```python
from build123d import *

# Parameters (mm, degrees)
SKETCH1_W            = 10.5
SKETCH1_H            = 6
BOSS_EXTRUDE1_DEPTH  = 7.07
SKETCH3_W            = 8.6
SKETCH3_H            = 1.8
CUT_EXTRUDE2_DEPTH   = 17
SKETCH4_W            = 10.5
SKETCH4_H            = 6
BOSS_EXTRUDE2_DEPTH  = 7.07
SKETCH5_W            = 4
SKETCH5_H            = 1.8
CUT_EXTRUDE3_DEPTH   = 19
FILLET1_R            = 12
FILLET2_R            = 12
SKETCH19_W           = 10.5
SKETCH19_H           = 11
SKETCH19_W_2         = 4
SKETCH19_H_2         = 1.8
BOSS_EXTRUDE8_DEPTH  = 15
CUT_EXTRUDE8_DEPTH   = 14.5
SKETCH21_W           = 10.5
SKETCH21_H           = 15
BOSS_EXTRUDE9_DEPTH  = 1
CUT_EXTRUDE10_DEPTH  = 15
FILLET6_R            = 2
FILLET12_R           = 2
BOSS_EXTRUDE15_DEPTH = 13
FILLET15_R           = 2
FILLET16_R           = 2
FILLET17_R           = 2


with BuildPart() as part:
    # Sketch1 → Boss-Extrude1 (new body)
    with BuildSketch(Plane.XY):
        Rectangle(SKETCH1_W, SKETCH1_H)
    extrude(amount=BOSS_EXTRUDE1_DEPTH)

    # Sketch3 → Cut-Extrude2 (cut)
    with BuildSketch(Plane.XY.offset(7.07)):
        Rectangle(SKETCH3_W, SKETCH3_H)
    extrude(amount=-CUT_EXTRUDE2_DEPTH, mode=Mode.SUBTRACT)

    # Sketch4 → Boss-Extrude2 (add)
    with BuildSketch(Plane.XY.offset(7.07)):
        Rectangle(SKETCH4_W, SKETCH4_H)
    extrude(amount=BOSS_EXTRUDE2_DEPTH)

    # Sketch5 → Cut-Extrude3 (cut, symmetric)
    with BuildSketch(Plane.XY.offset(14.14)):
        Rectangle(SKETCH5_W, SKETCH5_H)
    extrude(amount=CUT_EXTRUDE3_DEPTH, both=True, mode=Mode.SUBTRACT)

    # Fillet1
    # the kernel refuses this fillet: 12 mm, written as the material it takes off along each edge
    with BuildSketch(Plane(origin=(2, -0.9, 7.07), x_dir=(1, 0, 0), z_dir=(0, 1, 0))) as fillet1_piece_1:
        with BuildLine():
            CenterArc((12, -7.064700984), FILLET1_R, 143.93341174, 36.06658826)
            Line((0, -7.064700984), (0, 0))
            Line((0, 0), (2.3, 0))
        make_face()
    extrude(amount=1.8, mode=Mode.SUBTRACT)

    # Fillet2
    # the kernel refuses this fillet: 12 mm, written as the material it takes off along each edge
    with BuildSketch(Plane(origin=(-2, 0.9, 7.07), x_dir=(0, 0, 1), z_dir=(0, -1, 0))) as fillet2_piece_1:
        with BuildLine():
            CenterArc((7.064700984, 12), FILLET2_R, 233.93341174, 36.06658826)
            Line((0, 2.3), (0, 0))
            Line((0, 0), (7.064700984, 0))
        make_face()
    extrude(amount=1.8, mode=Mode.SUBTRACT)

    # Sketch19 → Boss-Extrude8 (add)
    with BuildSketch(Plane.XY.offset(14.14)):
        Rectangle(SKETCH19_W, SKETCH19_H)
        Rectangle(SKETCH19_W_2, SKETCH19_H_2, mode=Mode.SUBTRACT)
    extrude(amount=BOSS_EXTRUDE8_DEPTH)

    # Sketch20 → Cut-Extrude8 (cut)
    with BuildSketch(Plane.XY.offset(29.14)):
        with BuildLine():
            Line((1.996194266, 2.5), (1.996194266, 3.60169129))
            Line((1.996194266, 3.60169129), (1.996194266, 5.301713665))
            Line((1.996194266, 5.301713665), (0.55, 5.301713665))
            Line((0.55, 5.301713665), (0.55, 5.5))
            Line((0.55, 5.5), (-0.55, 5.5))
            Line((-0.55, 5.5), (-0.55, 5.301713665))
            Line((-0.55, 5.301713665), (-2.002287503, 5.301713665))
            Line((-2.002287503, 5.301713665), (-2.002287503, 2.5))
            Line((-2.002287503, 2.5), (-2.5, 2.5))
            Line((-2.5, 2.5), (-2.5, -2.5))
            Line((-2.5, -2.5), (-2.002287503, -2.5))
            Line((-2.002287503, -2.5), (-2.002287503, -3.60169129))
            Line((-2.002287503, -3.60169129), (0, -3.60169129))
            Line((0, -3.60169129), (1.996194266, -3.60169129))
            Line((1.996194266, -3.60169129), (1.996194266, -2.5))
            Line((1.996194266, -2.5), (2.5, -2.5))
            ThreePointArc((2.5, -2.5), (3.720567772, 0), (2.5, 2.5))
            Line((2.5, 2.5), (1.996194266, 2.5))
        make_face()
    extrude(amount=-CUT_EXTRUDE8_DEPTH, mode=Mode.SUBTRACT)

    # Sketch21 → Boss-Extrude9 (add)
    with BuildSketch(Plane(origin=(0, 5.5, 0), x_dir=(1, 0, 0), z_dir=(0, 1, 0))):
        with Locations((0, -21.64)):
            Rectangle(SKETCH21_W, SKETCH21_H)
    extrude(amount=BOSS_EXTRUDE9_DEPTH)

    # Sketch22 → Cut-Extrude10 (cut)
    with BuildSketch(Plane.XY.offset(29.14)):
        Polygon((3.285102714, 3.046335485), (5.25, 3.046335485), (5.25, 5.593635507), (5.25, 6.5), (3.747361829, 6.5), (3.285102714, 6.5), (3.285102714, 3.836641371), align=None)
        Polygon((-5.25, 5.593635507), (-5.25, 3.046335485), (-4.265605325, 3.046335485), (-3.285102714, 3.046335485), (-3.285102714, 4.03485795), (-3.285102714, 5.593635507), (-3.285102714, 6.5), (-5.25, 6.5), align=None)
        with BuildLine():
            Line((-5.25, -3.5), (-5.25, -5.5))
            Line((-5.25, -5.5), (5.25, -5.5))
            Line((5.25, -5.5), (5.25, -3.5))
            ThreePointArc((5.25, -3.5), (4.53848024, -3.923585886), (3.747361829, -4.16816109))
            Line((3.747361829, -4.16816109), (-3.701400921, -4.16816109))
            ThreePointArc((-3.701400921, -4.16816109), (-4.521026788, -3.939133518), (-5.25, -3.5))
        make_face()
    extrude(amount=-CUT_EXTRUDE10_DEPTH, mode=Mode.SUBTRACT)

    # Fillet6
    # the kernel refuses this fillet: 2 mm, written as the material it takes off along each edge
    with BuildSketch(Plane(origin=(8.294369106, -4.16816109, 14.14), x_dir=(0, 1, 0), z_dir=(-1, 0, 0))) as fillet6_piece_1:
        with BuildLine():
            CenterArc((2, -1.818802911), FILLET6_R, 114.577232298, 65.422767702)
            Line((0, -1.818802911), (-0.04, -1.818802911))
            Line((-0.04, -1.818802911), (-0.04, 0))
            Line((-0.04, 0), (0, 0.04))
            ThreePointArc((0, 0.04), (0.584080545, 0.04), (1.151524312, 0.036376058))
            Line((1.151524312, 0.036376058), (1.16816109, 0))
        make_face()
    extrude(amount=16.542777304, mode=Mode.SUBTRACT)

    # Fillet12
    fillet12_edges = [part.edges().sort_by_distance(p)[0] for p in [
        (5.25, -3, 7.07),
        (-5.25, -3, 7.07),
        (-5.25, 3, 7.07),
        (5.25, 3, 7.07),
    ]]
    fillet(fillet12_edges, radius=FILLET12_R)

    # Sketch24 → Boss-Extrude15 (add)
    with BuildSketch(Plane.XY.offset(29.14)):
        with BuildLine():
            Line((-1.004242215, -4.5), (-1.004242215, -5.004164362))
            ThreePointArc((-1.004242215, -5.004164362), (-0.001088997, -5.990129828), (1.002064221, -5.004164362))
            Line((1.002064221, -5.004164362), (1.002064221, -4.16816109))
            Line((1.002064221, -4.16816109), (1.699607491, -4.16816109))
            Line((1.699607491, -4.16816109), (1.699607491, -5.004164362))
            ThreePointArc((1.699607491, -5.004164362), (-0.003424292, -6.590087757), (-1.706456074, -5.004164362))
            Line((-1.706456074, -5.004164362), (-1.706456074, -4.16816109))
            Line((-1.706456074, -4.16816109), (-1.004242215, -4.16816109))
            Line((-1.004242215, -4.16816109), (-1.004242215, -4.5))
        make_face()
    extrude(amount=-BOSS_EXTRUDE15_DEPTH)

    # Fillet15
    fillet15_edges = [part.edges().sort_by_distance(p)[0] for p in [
        (0, 6.5, 14.14),
        (-3.285102714, 6.5, 21.64),
        (3.285102714, 6.5, 21.64),
    ]]
    fillet(fillet15_edges, radius=FILLET15_R)

    # Fillet16
    # the kernel refuses this fillet: 2 mm, written as the material it takes off along each edge
    with BuildSketch(Plane(origin=(5.25, 3.046335485, 34.14), x_dir=(-1, 0, 0), z_dir=(0, 0, -1))) as fillet16_piece_1_section:
        with BuildLine():
            CenterArc((FILLET16_R, -FILLET16_R), FILLET16_R, 90, 90)
            Line((0, -FILLET16_R), (0, 0))
            Line((0, 0), (FILLET16_R, 0))
        make_face()
    fillet16_piece_1 = extrude(amount=25, mode=Mode.PRIVATE)
    fillet16_piece_1 = split(fillet16_piece_1, bisect_by=Plane(origin=(3.285102714, 3.046335485, 34.14), z_dir=(1, 0, 0)), keep=Keep.TOP, mode=Mode.PRIVATE)
    add(fillet16_piece_1, mode=Mode.SUBTRACT)

    # Fillet17
    # the kernel refuses this fillet: 2 mm, written as the material it takes off along each edge
    with BuildSketch(Plane(origin=(-5.25, 3.046335485, 34.14), x_dir=(1, 0, 0), z_dir=(0, 0, -1))) as fillet17_piece_1_section:
        with BuildLine():
            CenterArc((FILLET17_R, FILLET17_R), FILLET17_R, 180, 90)
            Line((0, FILLET17_R), (0, 0))
            Line((0, 0), (FILLET17_R, 0))
        make_face()
    fillet17_piece_1 = extrude(amount=25, mode=Mode.PRIVATE)
    fillet17_piece_1 = split(fillet17_piece_1, bisect_by=Plane(origin=(-3.285102714, 3.046335485, 34.14), z_dir=(-1, 0, 0)), keep=Keep.TOP, mode=Mode.PRIVATE)
    add(fillet17_piece_1, mode=Mode.SUBTRACT)


solid = part.part
```
The model under review builds one solid part; all positions refer to its coordinate system, in mm. A direction names the side the tool comes from. Round coordinates to 2 decimals unless told otherwise and drop trailing zeros. Write each loop counter-clockwise with the first axis right and the second up, starting at its lowest first coordinate (ties: lowest second). Pieces come first, ordered by that corner, then holes.
(1) We need section C-C on y = 4. Give the boundary of the cut face in (x, z).
(2) We need section A-A on y = 0. Give the boundary of the cut face in (x, z), and give its area (3 significant figures).
(3) Insertion check: pin 1 (3 mm diameter, centred on x = 1, y = -1, fed in from +Z); pin 2 (0.7 mm diameter, centred on x = 1.5, z = 22, fed in from -Y); pin 3 (5 mm diameter, centred on x = 2.5, z = 3, fed in from +Y). Each pin has a flat end and moves straight along its axis. Give the tip position at first contact, or say it passes through.
(4) We need section D-D on z = 16.75. Give the number of separate pieces and of enclosed holes in the cut face, and give its area (3 significant figures).
(5) Mouldability with a two-part tool opening along X and no side actions: class faces 1 (the flat face through (0, 3, 7)), 2 (the flat face through (-1.004, -4.6, 22.7)), 3 (the cylindrical face through (0.03, -6.59, 22.73)) as +X half, -X half, draft (parallel to the pull), parting line (faces both ways), or undercut.
(6) Machinability: for faces 4 (the flat face through (0, -6.2, 16.14)), 5 (the cylindrical face through (-2.606, 0.013, 10.37)), 6 (the flat face through (3.285, 4, 22)), 7 (the cylindrical face through (-0.02, -5.99, 22.73)), 8 (the flat face through (-2.5, 0, 22)), which of the approach directions +Z, -Z, +X, -X, +Y, -Y give a long, thin tool a straight path to every point of the face, cutting with its end or side? Answer none if there is none.
(7) We need section B-B on z = 6.25. Give the boundary of the cut face in (x, y), and give its area (3 significant figures).
(8) Wall thickness on L1, parallel to X at y = -4.25, z = 18.5; L2, parallel to Y at x = 1.25, z = 12.5; L3, parallel to X at y = -3.25, z = 20.5: over which ranges is each line inside the solid? List them lowest first.
Findings below:
1. outline: (-3.29, 14.14) - (3.29, 14.14) - (3.29, 29.14) - (2, 29.14) - (2, 14.64) - (-2, 14.64) - (-2, 29.14) - (-3.29, 29.14) - close
2. outline: (-5.25, 0) - (-4.3, 0) - (-4.3, 7.07) arc R12 ccw to (-2, 14.13) - (-2, 14.64) - (-2.5, 14.64) - (-2.5, 29.14) - (-5.25, 29.14) - close; (2, 14.13) arc R12 ccw to (4.3, 7.07) - (4.3, 0) - (5.25, 0) - (5.25, 29.14) - (3.72, 29.14) - (3.72, 14.64) - (2, 14.64) - close
2. area: 114 mm2
3. pin 1: stops at z = 14.64
3. pin 2: stops at y = -6.14
3. pin 3: stops at y = 3
4. separate pieces: 1
4. enclosed holes: 2
4. area: 52.9 mm2
5. face 1: draft
5. face 2: undercut
5. face 3: parting line
6. face 4: -Z, +X, -X, -Y
6. face 5: -Z
6. face 6: +Z, -Z, +X, +Y
6. face 7: +Z, -Z
6. face 8: +Z
7. outline: (-5.25, -1) arc R2 ccw to (-3.25, -3) - (3.25, -3) arc R2 ccw to (5.25, -1) - (5.25, 1) arc R2 ccw to (3.25, 3) - (-3.25, 3) arc R2 ccw to (-5.25, 1) - close; hole (-4.3, -0.9) - (4.3, -0.9) - (4.3, 0.9) - (-4.3, 0.9) - close
7. area: 44.1 mm2
8. L1: x = -1.71 to -1, 1 to 1.7
8. L2: y = -3 to -0.9, 0.9 to 3
8. L3: x = -5.25 to -2, 2 to 5.25
